Geometry: see drawing. Coordinates: mm, zero at the bounding-box minimum. A direction names the side the tool comes from. Give positions to 0.01 mm unless a question says otherwise; leave off trailing zeros. Write each loop counter-clockwise with the first axis right and the second up, starting at its lowest first coordinate (ties: lowest second). Pieces come first, ordered by that corner, then holes. Notation, with made-up numbers: (77, 40) - (133, 40) arc R23 ccw to (133, 74) - close; hole circle Ø11 at (-9, 66.25). An arc over 180 degrees is marked (long way). Return JSON: item names as keys, results as strings.
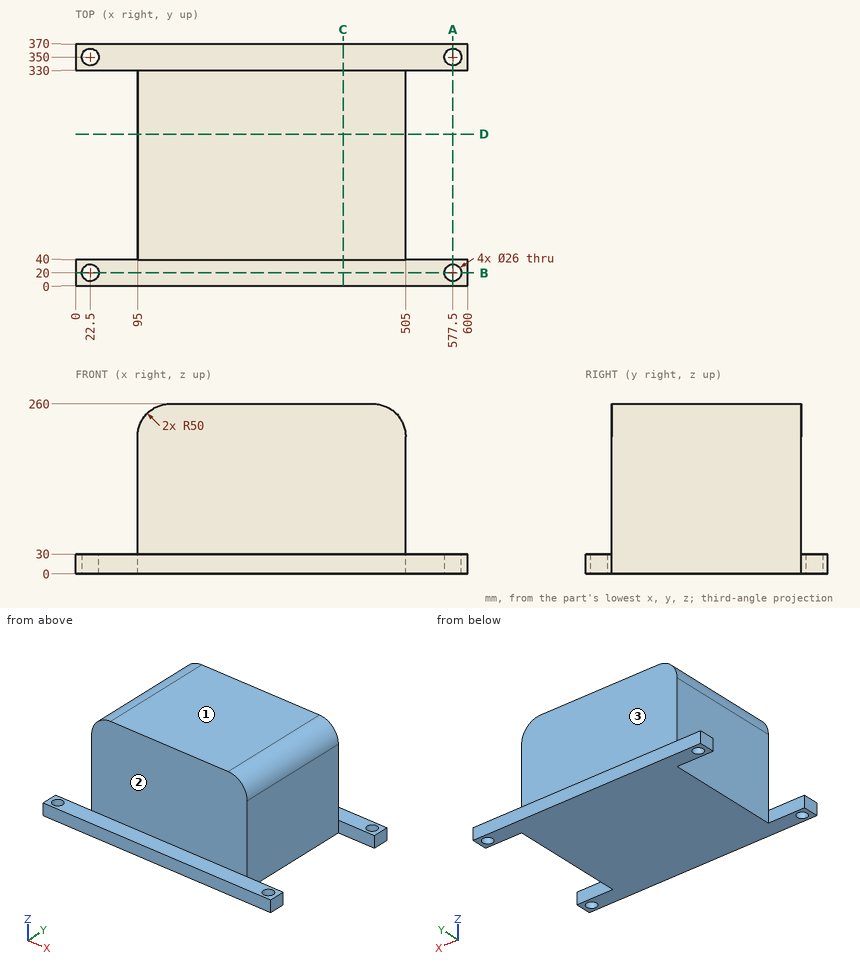
Q1. Material intervals for probe 1 along Y at (x, z) = (22.5, 20.75); probe 2 along X at (y, z) = (20, 14); probe 3 along X at (y, z) = (81, 146), sorted ascending. Write a range as [from, to].
Answer key:
{"probe 1": "y = [0, 7], [33, 40], [330, 337], [363, 370]", "probe 2": "x = [0, 9.5], [35.5, 564.5], [590.5, 600]", "probe 3": "x = [95, 505]"}
Q2. Set-up query: the marked faces 1, 2 and 3. Return all of +Z, -Z, +X, -X, +Y, -Y with unobstructed straight access to the full face (end or side cutting, diameter ignored); none if empty.
Answer key:
{"face 1": "+Z, +X, -X, +Y, -Y", "face 2": "+Z, +X, -X, -Y", "face 3": "+Z, +X, -X, +Y"}
Q3. Section query B-B, the plane y = 20. Return the cut outline in (x, z).
Answer key:
{"outline": "(0, 0) - (9.5, 0) - (9.5, 30) - (0, 30) - close; (35.5, 0) - (564.5, 0) - (564.5, 30) - (35.5, 30) - close; (590.5, 0) - (600, 0) - (600, 30) - (590.5, 30) - close"}
Q4. Pin query (flat end, axial travel): P1, Ø6, axis at y = 101, z = 135.5, coming from the -X side; P2, Ø8, axis at x = 145, z = 192.5, coming from the -Y side; P3, Ø20, axis at x = 423, y = 19, coming from the +Z side; P4, Ø21, axis at x = 577.5, y = 350, coming from the +Z side. Return the tip coordinate at first contact, or that it passes through.
Answer key:
{"P1": "stops at x = 95", "P2": "stops at y = 40", "P3": "stops at z = 30", "P4": "passes through"}
Q5. Section query A-A, the plane x = 577.5. Return the cut outline in (y, z).
Answer key:
{"outline": "(0, 0) - (7, 0) - (7, 30) - (0, 30) - close; (33, 0) - (40, 0) - (40, 30) - (33, 30) - close; (330, 0) - (337, 0) - (337, 30) - (330, 30) - close; (363, 0) - (370, 0) - (370, 30) - (363, 30) - close"}
Q6. Section query C-C, the plane x = 409.5. Return the cut outline in (y, z).
Answer key:
{"outline": "(0, 0) - (370, 0) - (370, 30) - (330, 30) - (330, 260) - (40, 260) - (40, 30) - (0, 30) - close"}
Q7. Section query D-D, the plane y = 232. Return the cut outline in (x, z), plus the area to 3 significant figures.
Answer key:
{"outline": "(95, 0) - (505, 0) - (505, 210) arc R50 ccw to (455, 260) - (145, 260) arc R50 ccw to (95, 210) - close", "area": "106,000 mm^2"}
